Can you work these out from the model? Positions are in its coordinate system, mm. Face numbers are marked on the shaded views. A direction names the side the tool comes from. Coordinates: 2 decimals unless noted, no trailing zeros. Loops run counter-clockwise (first coordinate to the right, second up) from the corner with the lowest first, then second, coordinate; pieces in that order, holes last. Notation, with made-up numbers: (28.5, 75.5) -> (73.5, 75.5) arc R24 cw to (73.5, 90.5) -> close; hole circle Ø8 at (-37, -3.5). An arc over 180 degrees is marked (long way). Use one line per item in the form item = value. Start each with the question number.
(1) On a 3-axis mill with a long thin cutter (end or side, diameter ignored), from which of +Z, -Z, +X, -X, +Y, -Y can I reach the whole of each face in a straight line? I mean the marked faces 1 and 2. Say none if no direction works.
(2) Imagine slicing it at A-A (y = 0). List the corners of the cut face in (x, z) for me.
(3) Imagine slicing it at C-C (x = -6.5). List the corners of the cut face in (y, z) for me.
(4) I'm going to push flat-ended pins straight in: pin 1 (8 mm diameter, centred on x = 24, z = 3, fed in from +Y); pin 2 (1.5 mm diameter, centred on x = 7.5, y = 0.5, fed in from +Z); pin 3 (2 mm diameter, centred on x = -3.5, y = 3.5, fed in from +Z). Where does each tip first touch, or does it pass through?
(5) I need wall thicknesses on line 1 (X direction, y = 5.5, z = -2.5); line 2 (X direction, y = -3, z = -1.25); line 3 (Z direction, x = -8, y = 0.25). Which ranges of each line are inside material? Lowest first, please. Write a range as [from, to].
(6) Imagine slicing it at D-D (z = -3.5). List the corners of the cut face in (x, y) for me, plus the area to 3 significant figures.
```python
from build123d import *

# Parameters (mm, degrees)
SKETCH1_R           = 5.5
BOSS_EXTRUDE2_DEPTH = 23.8
SKETCH2_R           = 7.2
BOSS_EXTRUDE4_DEPTH = 10.3
SKETCH3_R           = 2.5
BOSS_EXTRUDE5_DEPTH = 5


with BuildPart() as part:
    # Sketch1 → Boss-Extrude2 (new body)
    with BuildSketch(Plane(origin=(0, 0, 0), x_dir=(0, 0, -1), z_dir=(1, 0, 0))):
        Circle(SKETCH1_R)
    extrude(amount=BOSS_EXTRUDE2_DEPTH)

    # Sketch2 → Boss-Extrude4 (add)
    with BuildSketch(Plane.ZY):
        Circle(SKETCH2_R)
    extrude(amount=BOSS_EXTRUDE4_DEPTH)

    # Sketch3 → Boss-Extrude5 (add)
    with BuildSketch(Plane(origin=(23.8, 0, 0), x_dir=(0, 0, -1), z_dir=(1, 0, 0))):
        Circle(SKETCH3_R)
    extrude(amount=BOSS_EXTRUDE5_DEPTH)


solid = part.part
```
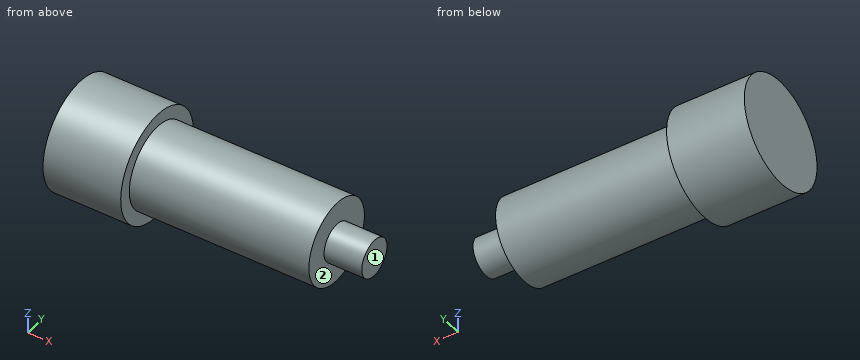
Worked out:
q1.face_1 = +Z, -Z, +X, +Y, -Y
q1.face_2 = +X
q2.outline = (-10.3, -7.2) -> (0, -7.2) -> (0, -5.5) -> (23.8, -5.5) -> (23.8, -2.5) -> (28.8, -2.5) -> (28.8, 2.5) -> (23.8, 2.5) -> (23.8, 5.5) -> (0, 5.5) -> (0, 7.2) -> (-10.3, 7.2) -> close
q3.outline = circle Ø14.4 at (0, 0)
q4.pin_1 = 5.5
q4.pin_2 = 5.5
q4.pin_3 = 6.75
q5.line_1 = [-10.3, 0]
q5.line_2 = [-10.3, 23.8]
q5.line_3 = [-7.2, 7.2]
q6.outline = (-10.3, -6.29) -> (0, -6.29) -> (0, -4.24) -> (23.8, -4.24) -> (23.8, 4.24) -> (0, 4.24) -> (0, 6.29) -> (-10.3, 6.29) -> close
q6.area = 332 mm2
